```python
from build123d import *

# Parameters (mm, degrees)
DRAFT_2_R           = 1.5
EXTRUDE_1_DEPTH     = 3
EXTRUDE_START       = -5
EXTRUDE_2_DEPTH     = 5
DRAFT_6_R           = 1.75
CUT_EXTRUDE_7_DEPTH = 64.227785822


with BuildPart() as part:
    # draft 2 → Extrude 1 (new body)
    with BuildSketch(Plane.XY):
        with BuildLine():
            Line((41.27, 36.8), (36.034054446, 36.8))
            Line((36.034054446, 36.8), (36.039162942, 39.737383337))
            ThreePointArc((36.039162942, 39.737383337), (33.044384867, 42.742596187), (30.039172016, 39.747818111))
            Line((30.039172016, 39.747818111), (30.034045372, 36.8))
            Line((30.034045372, 36.8), (-29.97, 36.8))
            Line((-29.97, 36.8), (-29.97, 39.8))
            ThreePointArc((-29.97, 39.8), (-32.97, 42.8), (-35.97, 39.8))
            Line((-35.97, 39.8), (-35.97, 36.8))
            Line((-35.97, 36.8), (-41.27, 36.8))
            ThreePointArc((-41.27, 36.8), (-44.805533906, 35.335533906), (-46.27, 31.8))
            Line((-46.27, 31.8), (-46.27, -31.8))
            ThreePointArc((-46.27, -31.8), (-44.805533906, -35.335533906), (-41.27, -36.8))
            Line((-41.27, -36.8), (-35.97, -36.8))
            Line((-35.97, -36.8), (-35.97, -39.8))
            ThreePointArc((-35.97, -39.8), (-32.97, -42.8), (-29.97, -39.8))
            Line((-29.97, -39.8), (-29.97, -36.8))
            Line((-29.97, -36.8), (30.034045372, -36.8))
            Line((30.034045372, -36.8), (30.039172016, -39.747818111))
            ThreePointArc((30.039172016, -39.747818111), (33.044384867, -42.742596187), (36.039162942, -39.737383337))
            Line((36.039162942, -39.737383337), (36.034054446, -36.8))
            Line((36.034054446, -36.8), (41.27, -36.8))
            ThreePointArc((41.27, -36.8), (44.805533906, -35.335533906), (46.27, -31.8))
            Line((46.27, -31.8), (46.27, 31.8))
            ThreePointArc((46.27, 31.8), (44.805533906, 35.335533906), (41.27, 36.8))
        make_face()
        with Locations((-32.97, -39.8)):
            Circle(DRAFT_2_R, mode=Mode.SUBTRACT)
        with Locations((33.039167479, -39.742600724)):
            Circle(DRAFT_2_R, mode=Mode.SUBTRACT)
        with Locations((-32.97, 39.8)):
            Circle(DRAFT_2_R, mode=Mode.SUBTRACT)
        with Locations((33.039167479, 39.742600724)):
            Circle(DRAFT_2_R, mode=Mode.SUBTRACT)
    extrude(amount=EXTRUDE_1_DEPTH)

    # draft_5 → Extrude 2 (add)
    with BuildSketch(Plane.XY.offset(EXTRUDE_START)):
        with BuildLine():
            ThreePointArc((-46.27, -31.8), (-44.805533906, -35.335533906), (-41.27, -36.8))
            Line((-41.27, -36.8), (-35.97, -36.8))
            Line((-35.97, -36.8), (-32.97, -36.8))
            Line((-32.97, -36.8), (-29.97, -36.8))
            Line((-29.97, -36.8), (30.034045372, -36.8))
            Line((30.034045372, -36.8), (32.455128971, -36.8))
            ThreePointArc((32.455128971, -36.8), (33.039167479, -36.742600724), (33.623205988, -36.8))
            Line((33.623205988, -36.8), (36.034054446, -36.8))
            Line((36.034054446, -36.8), (41.27, -36.8))
            ThreePointArc((41.27, -36.8), (44.805533906, -35.335533906), (46.27, -31.8))
            Line((46.27, -31.8), (46.27, 31.8))
            ThreePointArc((46.27, 31.8), (44.805533906, 35.335533906), (41.27, 36.8))
            Line((41.27, 36.8), (36.034054446, 36.8))
            Line((36.034054446, 36.8), (33.623205988, 36.8))
            ThreePointArc((33.623205988, 36.8), (33.039167479, 36.742600724), (32.455128971, 36.8))
            Line((32.455128971, 36.8), (30.034045372, 36.8))
            Line((30.034045372, 36.8), (-29.97, 36.8))
            Line((-29.97, 36.8), (-32.97, 36.8))
            Line((-32.97, 36.8), (-35.97, 36.8))
            Line((-35.97, 36.8), (-41.27, 36.8))
            ThreePointArc((-41.27, 36.8), (-44.805533906, 35.335533906), (-46.27, 31.8))
            Line((-46.27, 31.8), (-46.27, -31.8))
        make_face()
        Polygon((-44.27, 29.8), (-39.27, 34.8), (39.33, 34.8), (44.33, 29.8), (44.33, -29.8), (39.33, -34.8), (-39.27, -34.8), (-44.27, -29.8), align=None, mode=Mode.SUBTRACT)
    extrude(amount=EXTRUDE_2_DEPTH)

    # draft_6 → Cut-Extrude 7 (cut, through all)
    with BuildSketch(Plane.XY):
        with Locations((-32.97, 27)):
            Circle(DRAFT_6_R)
        with Locations((-32.97, -27)):
            Circle(DRAFT_6_R)
        with Locations((32.922993654, -27.057298255)):
            Circle(DRAFT_6_R)
        with Locations((33.016906626, 26.942620081)):
            Circle(DRAFT_6_R)
    extrude(amount=CUT_EXTRUDE_7_DEPTH, mode=Mode.SUBTRACT)


solid = part.part
```
Part model, mm, in its own coordinate system. A direction names the side the tool comes from. Round coordinates to 2 decimals unless told otherwise and drop trailing zeros. Loops run counter-clockwise (first coordinate to the right, second up) from the corner with the lowest first, then second, coordinate; pieces in that order, holes last.
1. Two-plate mould, pull along X, no slides. Class faces 1 (the face through (-35.97, -38, 1)), 2 (the face through (-4, 36.8, -1)), 3 (the face through (-34, -38, 0)): pulls with the +X half, pulls with the -X half, needs draft (parallel to the pull), parting line crosses it, or undercut.
Solutions:
face 1: pulls with the -X half
face 2: undercut
face 3: needs draft
2. 3-axis set-ups, long thin cutter, end or side, ignore diameter. For faces 4 (the face through (-35.97, 38, 1)), 5 (the face through (1, -34.8, -3)), 6 (the face through (-29.97, 38, 1)): which of +Z, -Z, +X, -X, +Y, -Y reach the whole face in a straight line?
Solutions:
face 4: +Z, -Z, -X, +Y
face 5: -Z
face 6: +Z, -Z, +Y
3. Flat gauge pins, fed straight in: pin 1 (3 mm diameter, centred on x = 34, y = -40, fed in from -Z); pin 2 (4 mm diameter, centred on x = 37.5, z = -2.5, fed in from +Y); pin 3 (3 mm diameter, centred on x = 29, z = 0.5, fed in from -Y). Where does each tip first touch, or does it go through?
Solutions:
pin 1: stops at z = 0
pin 2: stops at y = 36.8
pin 3: stops at y = -41.34
4. Drill centre lines: line 1 along X through (y, z) = (-27, 1.3); line 2 along Y through (x, z) = (3, -2); line 3 along X through (y, z) = (-12, -2.25). Where is each one in solid material? Low to high.
Solutions:
line 1: x = -46.27 to -34.72, -31.22 to 31.17, 34.67 to 46.27
line 2: y = -36.8 to -34.8, 34.8 to 36.8
line 3: x = -46.27 to -44.27, 44.33 to 46.27
5. Slice it at B-B (y = -10). Give the cut face in (x, z), and give its area (3 significant figures).
Solutions:
outline: (-46.27, -5) - (-44.27, -5) - (-44.27, 0) - (44.33, 0) - (44.33, -5) - (46.27, -5) - (46.27, 3) - (-46.27, 3) - close
area: 297 mm2
6. Slice it at A-A (x = 13.5). Give the cut face in (y, z).
Solutions:
outline: (-36.8, -5) - (-34.8, -5) - (-34.8, 0) - (34.8, 0) - (34.8, -5) - (36.8, -5) - (36.8, 3) - (-36.8, 3) - close
